Check sheet for the modelled part. Datum: model origin and axes. Units: mm. Face numbers are marked on the shaded views. A direction names the side the tool comes from. Give positions to 0.01 mm unless a question says otherwise; leave off trailing zeros. Loops run counter-clockwise (first coordinate to the right, second up) from the corner with the lowest first, then second, coordinate; pieces in that order, holes last.
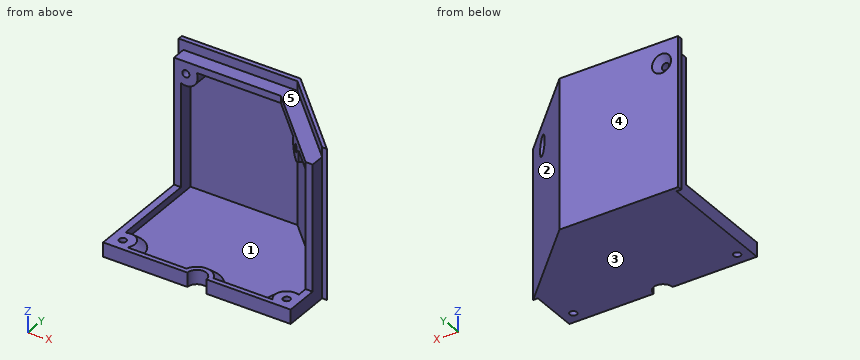
```python
from build123d import *
from OCP.BRepFilletAPI import BRepFilletAPI_MakeChamfer
from build123d.topology import SkipClean

# Parameters (mm, degrees)
EXTRUDE_1_DEPTH          = 63
EXTRUDE_2_DEPTH          = 3
SKETCH_3_W               = 3
SKETCH_3_H               = 6
EXTRUDE_3_DEPTH          = 56
EXTRUDE_4_DEPTH          = 3
SKETCH_6_W               = 3
SKETCH_6_H               = 6
EXTRUDE_5_DEPTH          = 45
SKETCH_7_W               = 3
SKETCH_7_H               = 6
EXTRUDE_6_DEPTH          = 14
SKETCH_8_R               = 4
CUT_EXTRUDE_1_DEPTH      = 3
EXTRUDE_7_DEPTH          = 3
SKETCH_10_R              = 5
EXTRUDE_8_DEPTH          = 3
SKETCH_12_R              = 5
EXTRUDE_9_DEPTH          = 6
CUT_EXTRUDE_3_DEPTH      = 113.049096382
CUT_EXTRUDE_3_DEPTH_BACK = 113.049096382
SKETCH_13_R              = 1.5
CHAMFER_2_SIZE           = 2.5
SKETCH_14_R              = 5
EXTRUDE_10_DEPTH         = 6.363961031
CUT_EXTRUDE_4_DEPTH      = 106.959898075
CUT_EXTRUDE_4_DEPTH_BACK = 106.959898075
SKETCH_15_R              = 1.5
CHAMFER_3_SIZE           = 2.5
CUT_EXTRUDE_5_DEPTH      = 105.398275848
CUT_EXTRUDE_5_DEPTH_BACK = 105.398275848
SKETCH_11_R              = 1.5
CHAMFER_4_SIZE           = 3
CHAMFER_4_SIZE_2         = 3.575260778


with BuildPart() as part:
    # Эскиз1 → Бобышка-Вытянуть1 (new body)
    with BuildSketch(Plane.XY):
        Polygon((0, 0), (-31, 31), (-81, 31), (-81, 33), (-31, 33), (2, 0), align=None)
    extrude(amount=EXTRUDE_1_DEPTH)

    # Эскиз2 → Бобышка-Вытянуть2 (add)
    with BuildSketch(Plane(origin=(0, 0, 0), x_dir=(-1, 0, 0), z_dir=(0, 0, -1))):
        Polygon((0, 0), (31, 31), (79, 31), (79, -20), (0, -20), align=None)
    extrude(amount=-EXTRUDE_2_DEPTH)

    # Эскиз3 → Бобышка-Вытянуть3 (add)
    with BuildSketch(Plane.XY.offset(3)):
        Polygon((0, 0), (0, -6), (-3, -6), (-3, 3), align=None)
        with Locations((-77.5, 28)):
            Rectangle(SKETCH_3_W, SKETCH_3_H)
    extrude(amount=EXTRUDE_3_DEPTH)

    # Эскиз5 → Бобышка-Вытянуть4 (add)
    with BuildSketch(Plane.XY.offset(59)):
        Polygon((-79, 25), (-76, 25), (-34, 25), (-3, -6), (0, -6), (0, 0), (-31, 31), (-79, 31), align=None)
    extrude(amount=-EXTRUDE_4_DEPTH)

    # Эскиз6 → Бобышка-Вытянуть5 (add)
    with BuildSketch(Plane.XZ.offset(-25)):
        with Locations((-77.5, 3)):
            Rectangle(SKETCH_6_W, SKETCH_6_H)
    extrude(amount=EXTRUDE_5_DEPTH)

    # Эскиз7 → Бобышка-Вытянуть6 (add)
    with BuildSketch(Plane.XZ.offset(6)):
        with Locations((-1.5, 3)):
            Rectangle(SKETCH_7_W, SKETCH_7_H)
    extrude(amount=EXTRUDE_6_DEPTH)

    # Эскиз8 → Вырез-Вытянуть1 (cut)
    with BuildSketch(Plane(origin=(0, 0, 0), x_dir=(-1, 0, 0), z_dir=(0, 0, -1))):
        with Locations((39.5, -20)):
            Circle(SKETCH_8_R)
    extrude(amount=-CUT_EXTRUDE_1_DEPTH, mode=Mode.SUBTRACT)

    # Эскиз9 → Бобышка-Вытянуть7 (add)
    with SkipClean():  # the faces are left unmerged after this step: merging them gives an invalid solid
        with BuildSketch(Plane.XY.offset(3)):
            with BuildLine():
                Line((-3, -20), (-35.5, -20))
                ThreePointArc((-35.5, -20), (-39.5, -16), (-43.5, -20))
                Line((-43.5, -20), (-76, -20))
                Line((-76, -20), (-76, -18))
                Line((-76, -18), (-45.156854249, -18))
                ThreePointArc((-45.156854249, -18), (-39.5, -14), (-33.843145751, -18))
                Line((-33.843145751, -18), (-3, -18))
                Line((-3, -18), (-3, -20))
            make_face()
        extrude(amount=EXTRUDE_7_DEPTH)
    add(part.part.scale(1), mode=Mode.REPLACE)  # the faces are merged on a copy

    # Эскиз10 → Бобышка-Вытянуть8 (add)
    with BuildSketch(Plane.XY.offset(3)):
        with Locations((-74, -15)):
            Circle(SKETCH_10_R)
        with Locations((-5, -15)):
            Circle(SKETCH_10_R)
    extrude(amount=EXTRUDE_8_DEPTH)

    # Эскиз12 → Бобышка-Вытянуть9 (add)
    with BuildSketch(Plane.XZ.offset(-31)):
        with Locations((-74, 54)):
            Circle(SKETCH_12_R)
    extrude(amount=EXTRUDE_9_DEPTH)

    # Эскиз13 → Вырез-Вытянуть3 (cut, two sides: drawn at the far end of the back side and taken through both)
    with BuildSketch(Plane.XZ.offset(-25).offset(-CUT_EXTRUDE_3_DEPTH_BACK)):
        with Locations(Location((-74, 54, 0), (0, 0, 270))):
            Circle(SKETCH_13_R)
    extrude(amount=CUT_EXTRUDE_3_DEPTH + CUT_EXTRUDE_3_DEPTH_BACK, mode=Mode.SUBTRACT)

    # Фаска2
    chamfer_2_edges = [part.edges().sort_by_distance(p)[0] for p in [
        (-74, 33, 55.5),
    ]]
    chamfer(chamfer_2_edges, length=CHAMFER_2_SIZE)

    # Эскиз14 → Бобышка-Вытянуть10 (add)
    with BuildSketch(Plane(origin=(0, 0, 0), x_dir=(0, 0, 1), z_dir=(-0.7071067811865462, -0.7071067811865489, 0))):
        with Locations((54, 15)):
            Circle(SKETCH_14_R)
    extrude(amount=EXTRUDE_10_DEPTH)

    # Эскиз15 → Вырез-Вытянуть4 (cut, two sides: drawn at the far end of the back side and taken through both)
    with BuildSketch(Plane(origin=(-4.5, -4.5, 0), x_dir=(0, 0, 1), z_dir=(-0.7071067811865464, -0.7071067811865488, 0)).offset(-CUT_EXTRUDE_4_DEPTH_BACK)):
        with Locations(Location((54, 15, 0), (0, 0, 270))):
            Circle(SKETCH_15_R)
    extrude(amount=CUT_EXTRUDE_4_DEPTH + CUT_EXTRUDE_4_DEPTH_BACK, mode=Mode.SUBTRACT)

    # Фаска3
    chamfer_3_edges = [part.edges().sort_by_distance(p)[0] for p in [
        (-10.66726189, 12.66726189, 54),
    ]]
    chamfer(chamfer_3_edges, length=CHAMFER_3_SIZE)

    # Эскиз11 → Вырез-Вытянуть5 (cut, two sides: drawn at the far end of the back side and taken through both)
    with BuildSketch(Plane.XY.offset(6).offset(-CUT_EXTRUDE_5_DEPTH_BACK)):
        with Locations((-74, -15)):
            Circle(SKETCH_11_R)
        with Locations((-5, -15)):
            Circle(SKETCH_11_R)
    extrude(amount=CUT_EXTRUDE_5_DEPTH + CUT_EXTRUDE_5_DEPTH_BACK, mode=Mode.SUBTRACT)

    # Фаска4
    chamfer_4_edges_1 = [part.edges().sort_by_distance(p)[0] for p in [
        (-8.920951867, -11.897398437, 3),
    ]]
    chamfer_4_side_1 = [part.faces().sort_by_distance(p)[0] for p in [
        (-8.920951867, -11.897398437, 3.06),
    ]]
    chamfer_4_edges_2 = [part.edges().sort_by_distance(p)[0] for p in [
        (-70.079048133, -11.897398437, 3),
    ]]
    chamfer_4_side_2 = [part.faces().sort_by_distance(p)[0] for p in [
        (-70.079048133, -11.897398437, 3.06),
    ]]
    chamfer_4_edges_3 = [part.edges().sort_by_distance(p)[0] for p in [
        (-21.421572875, -18, 3),
    ]]
    chamfer_4_side_3 = [part.faces().sort_by_distance(p)[0] for p in [
        (-21.421572875, -18, 3.06),
    ]]
    chamfer_4_edges_4 = [part.edges().sort_by_distance(p)[0] for p in [
        (-39.5, -14, 3),
    ]]
    chamfer_4_side_4 = [part.faces().sort_by_distance(p)[0] for p in [
        (-39.5, -14, 3.06),
    ]]
    chamfer_4_edges_5 = [part.edges().sort_by_distance(p)[0] for p in [
        (-57.578427125, -18, 3),
    ]]
    chamfer_4_side_5 = [part.faces().sort_by_distance(p)[0] for p in [
        (-57.578427125, -18, 3.06),
    ]]
    chamfer_4 = BRepFilletAPI_MakeChamfer(part.part.solid().wrapped)
    for e in chamfer_4_edges_1:
        chamfer_4.Add(CHAMFER_4_SIZE - 0.0001, CHAMFER_4_SIZE_2 - 0.0001, e.wrapped, chamfer_4_side_1[0].wrapped)
    for e in chamfer_4_edges_2:
        chamfer_4.Add(CHAMFER_4_SIZE - 0.0001, CHAMFER_4_SIZE_2 - 0.0001, e.wrapped, chamfer_4_side_2[0].wrapped)
    for e in chamfer_4_edges_3:
        chamfer_4.Add(CHAMFER_4_SIZE - 0.0001, CHAMFER_4_SIZE_2 - 0.0001, e.wrapped, chamfer_4_side_3[0].wrapped)
    for e in chamfer_4_edges_4:
        chamfer_4.Add(CHAMFER_4_SIZE - 0.0001, CHAMFER_4_SIZE_2 - 0.0001, e.wrapped, chamfer_4_side_4[0].wrapped)
    for e in chamfer_4_edges_5:
        chamfer_4.Add(CHAMFER_4_SIZE - 0.0001, CHAMFER_4_SIZE_2 - 0.0001, e.wrapped, chamfer_4_side_5[0].wrapped)
    add(Compound.cast(chamfer_4.Shape()), mode=Mode.REPLACE)  # a hair under: the kernel refuses the full size


solid = part.part
```
(1) Section check B-B on y = 26. Record the boundary of the cut face in (x, z), plus the area to 3 significant figures.
(2) Release check for a two-part mould opening along X. For the marked faces 1, 2 and 3 record: pulls with the +X half, pulls with the -X half, needs draft (parallel to the pull), parting line crosses it, or undercut.
(3) Section check D-D on y = -3. Record the boundary of the cut face in (x, z).
(4) Section check C-C on z = 10. Record the boundary of the cut face in (x, y), plus the area to 4 significant figures.
(5) Gauge pin test, flat ends, axial feed: pin 1 Ø13.5 at (x, z) = (-46.5, 19.5) entering from -Y; pin 2 Ø12 at (x, y) = (-44, 24.5) entering from -Z; pin 3 Ø4 at (y, z) = (12, 43) entering from +X; pin 4 Ø3 at (x, z) = (-6.5, 20.5) entering from -Y. Record the tip position at first contact, or that the pin passes through.
(6) Access from +Z, -Z, +X, -X, +Y, -Y to the whole of each face (thin tool, end or side, straight path). Record for the marked faces 4 and 5.
(7) Material ranges on line 1 (Z direction, x = -74, y = 27.05); line 2 (Y direction, x = -5, z = 4); line 3 (Y direction, x = -74, z = 1.35), recorded low to high.
Computed values:
1. outline: (-79, 0) - (-24, 0) - (-24, 63) - (-26, 63) - (-26, 59) - (-79, 59) - close; hole (-76, 3) - (-26, 3) - (-26, 56) - (-69.42, 56) arc R5 cw to (-76, 49.42) - close; hole circle Ø3 at (-74, 54)
1. area: 639 mm2
2. face 1: undercut
2. face 2: pulls with the +X half
2. face 3: needs draft
3. outline: (-79, 0) - (0, 0) - (0, 59) - (-6, 59) - (-6, 56) - (-3, 56) - (-3, 3) - (-76, 3) - (-76, 6) - (-79, 6) - close
4. outline: (-81, 31) - (-79, 31) - (-79, 25) - (-76, 25) - (-76, 31) - (-31, 31) - (-3, 3) - (-3, -6) - (0, -6) - (0, 0) - (2, 0) - (-31, 33) - (-81, 33) - close
4. area: 204.5 mm2
5. pin 1: stops at y = 31
5. pin 2: stops at z = 0
5. pin 3: stops at x = -8
5. pin 4: stops at y = 5
6. face 4: +Z, -Z, +X, -X, +Y
6. face 5: +Z, -X, -Y
7. line 1: z = 0 to 3, 49 to 52.5, 55.5 to 59
7. line 2: y = -20 to -16.5, -13.5 to -7.62, 5 to 7
7. line 3: y = -20 to -16.5, -13.5 to 33
